Autodesk Inventor part; units mm, degrees
ref_plane "YZ Plane" through (0, 0, 0) normal (1, 0, 0) x (0, 1, 0)
ref_plane "XZ Plane" through (0, 0, 0) normal (0, 1, 0) x (-1, 0, 0)
ref_plane "XY Plane" through (0, 0, 0) normal (0, 0, 1) x (1, 0, 0)
sketch "Sketch1" plane through (0, 0, 0) normal (0, 0, 1) x (1, 0, 0)
  line L0 (0, 0) -> (19.05, 0)
  line L1 (0, 0) -> (19.05, 0) construction
  line L2 (19.05, 0) -> (19.05, 82.55)
  line L3 (19.05, 82.55) -> (15.875, 82.55)
  line L4 (15.875, 82.55) -> (15.875, 3.175)
  line L5 (15.875, 3.175) -> (0, 3.175)
  line L6 (0, 3.175) -> (0, 0)
  dimension "d0" = 19.05
  dimension "d1" = 0
  dimension "d2" = 82.55
  dimension "d3" = 90
  dimension "d4" = 3.175
  dimension "d5" = 79.375
sketch "Sketch2" plane through (0, 0, 0) normal (0, 0, 1) x (1, 0, 0)
  point P0 (0, 0)
extrude "Extrusion3" add sketch "Sketch1" along normal blind 809.625
properties part number "ISPFrame"
Design review of the part built by this model. Coordinates are the model's own, in mm. A direction names the side the tool comes from. Give positions to 0.01 mm unless a question says otherwise; leave off trailing zeros. Loops run counter-clockwise (first coordinate to the right, second up) from the corner with the lowest first, then second, coordinate; pieces in that order, holes last. Notation, with made-up numbers: M 1,55.25 L 34,55.25 A21 cw 34,93.25 Z; hole C 62,72.5 d1. An arc over 180 degrees is marked long. Return JSON: item names as keys, results as strings. Group by question number.
Item 1: We need section A-A (z = 585.5). Give the boundary of the cut face in (x, y) (3 decimals).
Item 2: We need section B-B (x = 5). Give the boundary of the cut face in (y, z) (3 decimals), and give its area (3 significant figures).
Item 3: For probe 1 along X at (y, z) = (55.5, 358.5) (3 decimals); probe 2 along Y at (x, z) = (3.25, 418.5) (3 decimals), list the stretches that pass through material, from the lowest coordinate up.
Item 4: We need section C-C (y = 75.5). Give the boundary of the cut face in (x, z) (3 decimals), and give its area (3 significant figures).
Item 5: Tool access review of faces 1 (the flat face through (8, 3.175, 399)), 2 (the flat face through (17, 35, 0)): name each direction out of +Z, -Z, +X, -X, +Y, -Y from which nothing blocks a thin tool from reaching the whole face with its end or side.
Item 6: Insertion check: pin 1 Ø10 at (y, z) = (64.5, 433) entering from -X (3 decimals); pin 2 Ø2 at (x, y) = (17, 27) entering from -Z; pin 3 Ø1 at (x, z) = (10.5, 561) entering from +Y (3 decimals). Each pin has a flat end and moves straight along its axis. Give the tip position at first contact, or say it passes through.
Output:
{
 "1": {"outline": "M 0,0 L 19.05,0 L 19.05,82.55 L 15.875,82.55 L 15.875,3.175 L 0,3.175 Z"},
 "2": {"outline": "M 0,0 L 3.175,0 L 3.175,809.625 L 0,809.625 Z", "area": "2,570 mm^2"},
 "3": {"probe 1": "x = 15.875 to 19.05", "probe 2": "y = 0 to 3.175"},
 "4": {"outline": "M 15.875,0 L 19.05,0 L 19.05,809.625 L 15.875,809.625 Z", "area": "2,570 mm^2"},
 "5": {"face 1": "+Z, -Z, -X, +Y", "face 2": "-Z, +X, -X, +Y, -Y"},
 "6": {"pin 1": "stops at x = 15.875", "pin 2": "stops at z = 0", "pin 3": "stops at y = 3.175"}
}
